```python
from build123d import *

# Parameters (mm, degrees)
SKETCH1_W                      = 45
SKETCH1_H                      = 2350
BOSS_EXTRUDE1_DEPTH            = 31.5
SKETCH2_W                      = 6
SKETCH2_H                      = 2350
BOSS_EXTRUDE2_DEPTH            = 145
SKETCH3_W                      = 45
SKETCH3_H                      = 2350
BOSS_EXTRUDE3_DEPTH            = 76.5
SKETCH4_W                      = 6
SKETCH4_H                      = 2350
BOSS_EXTRUDE4_DEPTH            = 51
SKETCH5_W                      = 6
SKETCH5_H                      = 2350
BOSS_EXTRUDE5_DEPTH            = 24
SKETCH6_W                      = 15
SKETCH6_H                      = 2350
CUT_EXTRUDE1_DEPTH             = 6
SKETCH7_W                      = 39
SKETCH7_H                      = 2350
CUT_EXTRUDE2_DEPTH             = 45
SKETCH8_W                      = 100
SKETCH8_H                      = 6
CUT_EXTRUDE3_DEPTH             = 100
SKETCH9_W                      = 45
SKETCH9_H                      = 2350
BOSS_EXTRUDE6_DEPTH            = 25.5
SKETCH10_W                     = 39
SKETCH10_H                     = 51
CUT_EXTRUDE4_DEPTH             = 2351
SKETCH11_W                     = 6
SKETCH11_H                     = 2350
BOSS_EXTRUDE7_DEPTH            = 29
SKETCH12_W                     = 45
SKETCH12_H                     = 2350
BOSS_EXTRUDE8_DEPTH            = 25.5
SKETCH13_W                     = 39
SKETCH13_H                     = 51
CUT_EXTRUDE5_DEPTH             = 2351
SKETCH14_W                     = 6
SKETCH14_H                     = 2350
BOSS_EXTRUDE9_DEPTH            = 29
F_10_0_10_DIAMETER_HOLE1_D     = 10
F_10_0_10_DIAMETER_HOLE1_DEPTH = 6
F_10_0_10_DIAMETER_HOLE2_D     = 10
F_10_0_10_DIAMETER_HOLE2_DEPTH = 45
SKETCH24_W                     = 287.862467109
SKETCH24_H                     = 163.242221956
CUT_EXTRUDE8_DEPTH             = 800


with BuildPart() as part:
    # Sketch1 → Boss-Extrude1 (new body)
    with BuildSketch(Plane(origin=(0, 0, -76.5), x_dir=(-1, 0, 0), z_dir=(0, 0, -1))):
        with Locations((-72.5, 1175)):
            Rectangle(SKETCH1_W, SKETCH1_H)
    extrude(amount=-BOSS_EXTRUDE1_DEPTH)

    # Sketch2 → Boss-Extrude2 (add)
    with BuildSketch(Plane.ZY.offset(-50)):
        with Locations((-73.5, 1175)):
            Rectangle(SKETCH2_W, SKETCH2_H)
    extrude(amount=BOSS_EXTRUDE2_DEPTH)

    # Sketch3 → Boss-Extrude3 (add)
    with BuildSketch(Plane.XY.offset(-70.5)):
        with Locations((-72.5, 1175)):
            Rectangle(SKETCH3_W, SKETCH3_H)
    extrude(amount=BOSS_EXTRUDE3_DEPTH)

    # Sketch4 → Boss-Extrude4 (add)
    with BuildSketch(Plane.XY.offset(-45)):
        with Locations((92, 1175)):
            Rectangle(SKETCH4_W, SKETCH4_H)
    extrude(amount=BOSS_EXTRUDE4_DEPTH)

    # Sketch5 → Boss-Extrude5 (add)
    with BuildSketch(Plane.ZY.offset(-89)):
        with Locations((3, 1175)):
            Rectangle(SKETCH5_W, SKETCH5_H)
    extrude(amount=BOSS_EXTRUDE5_DEPTH)

    # Sketch6 → Cut-Extrude1 (cut)
    with BuildSketch(Plane.XY.offset(6)):
        with Locations((-57.5, 1175)):
            Rectangle(SKETCH6_W, SKETCH6_H)
    extrude(amount=-CUT_EXTRUDE1_DEPTH, mode=Mode.SUBTRACT)

    # Sketch7 → Cut-Extrude2 (cut)
    with BuildSketch(Plane.XY):
        with Locations((-69.5, 1175)):
            Rectangle(SKETCH7_W, SKETCH7_H)
    extrude(amount=-CUT_EXTRUDE2_DEPTH, mode=Mode.SUBTRACT)

    # Sketch8 → Cut-Extrude3 (cut)
    with BuildSketch(Plane(origin=(0, 2350, 0), x_dir=(-1, 0, 0), z_dir=(0, 1, 0))):
        with Locations((0, -73.5)):
            Rectangle(SKETCH8_W, SKETCH8_H)
    extrude(amount=-CUT_EXTRUDE3_DEPTH, mode=Mode.SUBTRACT)

    # Sketch9 → Boss-Extrude6 (add)
    with BuildSketch(Plane(origin=(0, 0, -76.5), x_dir=(-1, 0, 0), z_dir=(0, 0, -1))):
        with Locations((-72.5, 1175)):
            Rectangle(SKETCH9_W, SKETCH9_H)
    extrude(amount=BOSS_EXTRUDE6_DEPTH)

    # Sketch10 → Cut-Extrude4 (cut, through all)
    with BuildSketch(Plane.XZ):
        with Locations((75.5, -76.5)):
            Rectangle(SKETCH10_W, SKETCH10_H)
    extrude(amount=-CUT_EXTRUDE4_DEPTH, mode=Mode.SUBTRACT)

    # Sketch11 → Boss-Extrude7 (add)
    with BuildSketch(Plane(origin=(56, 0, 0), x_dir=(0, 0, -1), z_dir=(1, 0, 0))):
        with Locations((99, 1175)):
            Rectangle(SKETCH11_W, SKETCH11_H)
    extrude(amount=BOSS_EXTRUDE7_DEPTH)

    # Sketch12 → Boss-Extrude8 (add)
    with BuildSketch(Plane(origin=(0, 0, -76.5), x_dir=(-1, 0, 0), z_dir=(0, 0, -1))):
        with Locations((72.5, 1175)):
            Rectangle(SKETCH12_W, SKETCH12_H)
    extrude(amount=BOSS_EXTRUDE8_DEPTH)

    # Sketch13 → Cut-Extrude5 (cut, through all)
    with BuildSketch(Plane(origin=(0, 2350, 0), x_dir=(-1, 0, 0), z_dir=(0, 1, 0))):
        with Locations((75.5, -76.5)):
            Rectangle(SKETCH13_W, SKETCH13_H)
    extrude(amount=-CUT_EXTRUDE5_DEPTH, mode=Mode.SUBTRACT)

    # Sketch14 → Boss-Extrude9 (add)
    with BuildSketch(Plane.ZY.offset(56)):
        with Locations((-99, 1175)):
            Rectangle(SKETCH14_W, SKETCH14_H)
    extrude(amount=BOSS_EXTRUDE9_DEPTH)

    # Ø10.0 (10) Diameter Hole1
    with Locations(Plane.ZY.offset(56)):
        with Locations((-73.5, 2330)):
            Hole(F_10_0_10_DIAMETER_HOLE1_D / 2, depth=F_10_0_10_DIAMETER_HOLE1_DEPTH)

    # Ø10.0 (10) Diameter Hole2
    with Locations(Plane.ZY.offset(-50)):
        with Locations((-73.5, 2330)):
            Hole(F_10_0_10_DIAMETER_HOLE2_D / 2, depth=F_10_0_10_DIAMETER_HOLE2_DEPTH)

    # Sketch24 → Cut-Extrude8 (cut)
    with BuildSketch(Plane(origin=(0, 2350, 0), x_dir=(1, 0, 0), z_dir=(0, 1, 0))):
        with Locations((3.257138833, 40.584576945)):
            Rectangle(SKETCH24_W, SKETCH24_H)
    extrude(amount=-CUT_EXTRUDE8_DEPTH, mode=Mode.SUBTRACT)


solid = part.part
```
Model file for the job. Use its own axes, mm. A direction names the side the tool comes from. Give positions to 0.01 mm unless a question says otherwise; leave off trailing zeros. Write each loop counter-clockwise with the first axis right and the second up, starting at its lowest first coordinate (ties: lowest second). Pieces come first, ordered by that corner, then holes. Notation, with made-up numbers: (-25.5, 48.5) -> (-11.5, 48.5) arc R16 cw to (-11.5, 62.5) -> close; hole circle Ø5 at (54.5, 57.5). An arc over 180 degrees is marked (long way). Use CSV: the item, a comma, the result in double quotes. Start each with the question number.
1) Cut at C-C on x = -1. List the corners of the cut face in (y, z), plus the area to 3 significant figures.
2) Cut at B-B on y = 965. List the corners of the cut face in (x, z), plus the area to 3 significant figures.
3) Two-plate mould, pull along Z, no slides. Class faces 1 (the flat face through (50, 764, -58)), 2 (the flat face through (-89, 764, -22)), 3 (the flat face through (56, 764, -74)), 4 (the flat face through (1, 764, -70.5)): released by +Z, released by -Z, zero draft, split by the parting line, or undercut.
4) Drill centre lines: L1, parallel to Z at x = -68, y = 87; L2, parallel to X at y = 366, z = -13; L3, parallel to X at y = 199.5, z = -45.5. Where is each one in solid material? Low to high.
5) Tool access for faces 5 (the flat face through (75, 764, -51)), 6 (the flat face through (-50, 764, -58)), 7 (the flat face through (-75, 786, -51)), 8 (the flat face through (50, 764, -89)): list every direction of +Z, -Z, +X, -X, +Y, -Y with a clear straight run to the whole face (end or side of a thin tool).
6) Pin check, flat tips, straight feed: P1, Ø8.5, axis at x = -63.5, y = 974, coming from the +Z side; P2, Ø5, axis at y = 999.5, z = -100, coming from the -X side; P3, Ø12, axis at y = 648, z = -77, coming from the -X side; P4, Ø6, axis at x = 18.5, y = 1244.5, coming from the +Z side. Stop position of each tip, or through.
7) Cut at A-A on z = -29. List the corners of the cut face in (x, y).
Final values:
1,outline,"(0, -76.5) -> (1550, -76.5) -> (1550, -70.5) -> (0, -70.5) -> close"
1,area,"9,300 mm2"
2,outline,"(-95, -51) -> (-56, -51) -> (-56, -96) -> (-85, -96) -> (-85, -102) -> (-50, -102) -> (-50, -76.5) -> (50, -76.5) -> (50, -102) -> (85, -102) -> (85, -96) -> (56, -96) -> (56, -51) -> (95, -51) -> (95, 6) -> (65, 6) -> (65, 0) -> (89, 0) -> (89, -45) -> (50, -45) -> (50, -70.5) -> (-50, -70.5) -> (-50, -45) -> (-89, -45) -> (-89, 0) -> (-65, 0) -> (-65, 6) -> (-95, 6) -> close"
2,area,"3,000 mm2"
3,face 1,"zero draft"
3,face 2,"undercut"
3,face 3,"undercut"
3,face 4,"released by +Z"
4,L1,"z = -102 to -96, -51 to -45, 0 to 6"
4,L2,"x = -95 to -89, 89 to 95"
4,L3,"x = -95 to -50, 50 to 95"
5,face 5,"+X, +Y, -Y"
5,face 6,"+Z, +Y, -Y"
5,face 7,"-X, +Y, -Y"
5,face 8,"-Z, +Y, -Y"
6,P1,"stops at z = 6"
6,P2,"stops at x = -85"
6,P3,"stops at x = -56"
6,P4,"stops at z = -70.5"
7,outline,"(-95, 0) -> (-89, 0) -> (-89, 1550) -> (-95, 1550) -> close; (89, 0) -> (95, 0) -> (95, 1550) -> (89, 1550) -> close"
